Verification items for this drawing (mm, ordinates from the low corner). A direction names the side the tool comes from. Give positions to 0.01 mm unless a question says otherwise; leave off trailing zeros. Order: outer loops, then holes, each group sorted by start corner. A loop starts at its lowest first (then second) coordinate and runs counter-clockwise, first axis right, second up. Notation, with made-up numbers: (20.5, 49.25) -> (65.5, 49.25) arc R30 ccw to (65.5, 79.25) -> close; hole circle Ø10 at (45, -40). An arc over 180 degrees is marked (long way). One line per question, with ' | ' between items.
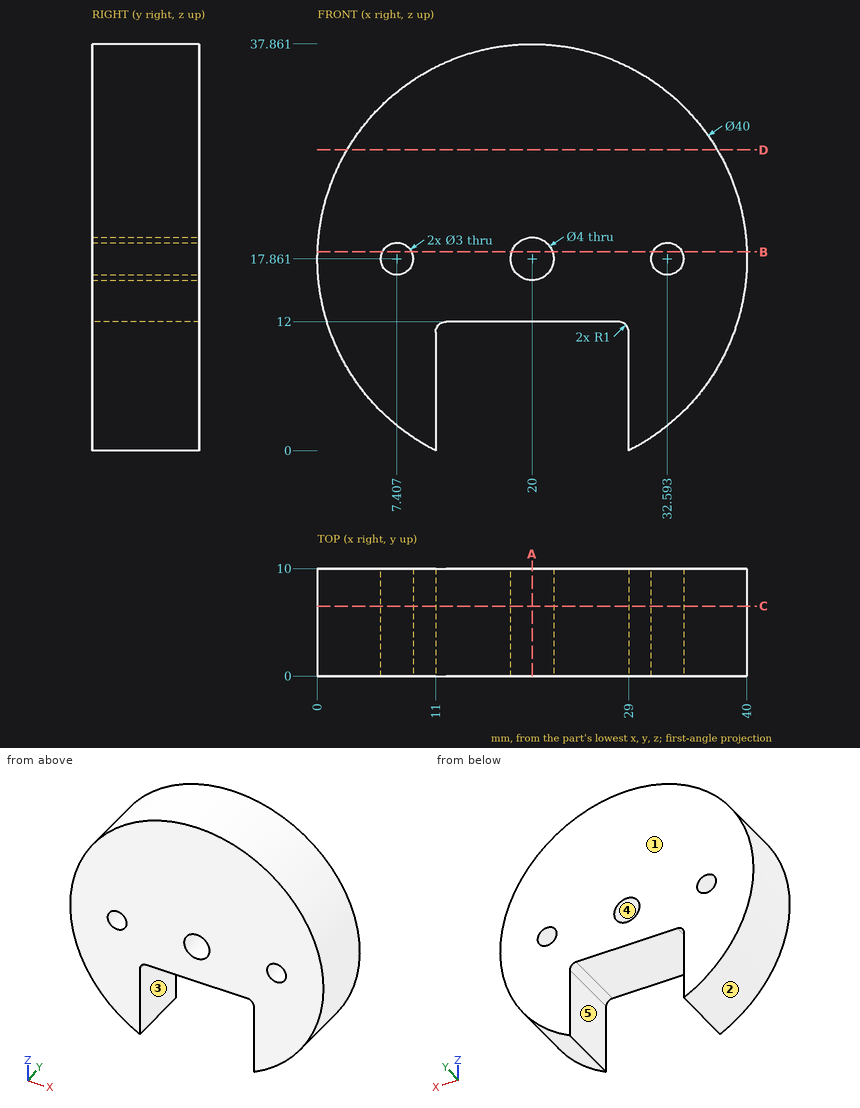
Q1. Access from +Z, -Z, +X, -X, +Y, -Y to the whole of each face (thin tool, end or side, straight path). Record for the marked faces 4 and 5.
Result sheet:
face 4: +Y, -Y | face 5: -Z, +Y, -Y
Q2. Section check A-A (x = 20). Enter the section's corners in (y, z).
Result sheet:
outline: (0, 12) -> (10, 12) -> (10, 15.86) -> (0, 15.86) -> close; (0, 19.86) -> (10, 19.86) -> (10, 37.86) -> (0, 37.86) -> close
Q3. Mould release check, pull along X, two halves, no side actions. Record for the marked faces 1, 2 and 3: pulls with the +X half, pulls with the -X half, needs draft (parallel to the pull), parting line crosses it, or undercut.
Result sheet:
face 1: needs draft | face 2: parting line crosses it | face 3: undercut
Q4. Section check C-C (y = 6.5). Enter the section's corners in (x, z).
Result sheet:
outline: (11, 0) -> (11, 11) arc R1 cw to (12, 12) -> (28, 12) arc R1 cw to (29, 11) -> (29, 0) arc R20 ccw (long way) to start; hole circle Ø3 at (7.41, 17.86); hole circle Ø4 at (20, 17.86); hole circle Ø3 at (32.59, 17.86)
Q5. Depth check by flat-ended pin: pin 1 Ø1 at (x, z) = (19.5, 18) entering from -Y; pin 2 Ø3 at (y, z) = (2.5, 4.5) entering from -X; pin 3 Ø5 at (y, z) = (3.5, 5) entering from +X; pin 4 Ø3 at (x, y) = (21, 8) entering from -Z. Enter the tip coordinate at first touch or a pass-through.
Result sheet:
pin 1: passes through | pin 2: stops at x = 3.9 | pin 3: stops at x = 37.11 | pin 4: stops at z = 12
Q6. Section check B-B (z = 18.5). Count the separate pieces of the cut face and the enclosed holes in it, and give its area (3 significant figures).
Result sheet:
separate pieces: 4 | enclosed holes: 0 | area: 308 mm2
Q7. Section check D-D (z = 28). Enter the section's corners in (x, y), and give its area (3 significant figures).
Result sheet:
outline: (2.76, 0) -> (37.24, 0) -> (37.24, 10) -> (2.76, 10) -> close | area: 345 mm2
Q8. Thickness scan on line 1 (Z direction, x = 20, y = 3); line 2 (X direction, y = 2.75, z = 6) (1 decimal); line 3 (X direction, y = 1.5, z = 8.5) (1 decimal). Record the ranges inside material, lowest first.
Result sheet:
line 1: z = 12 to 15.86, 19.86 to 37.86 | line 2: x = 3.9 to 11, 29 to 36.1 | line 3: x = 2.3 to 11, 29 to 37.7
